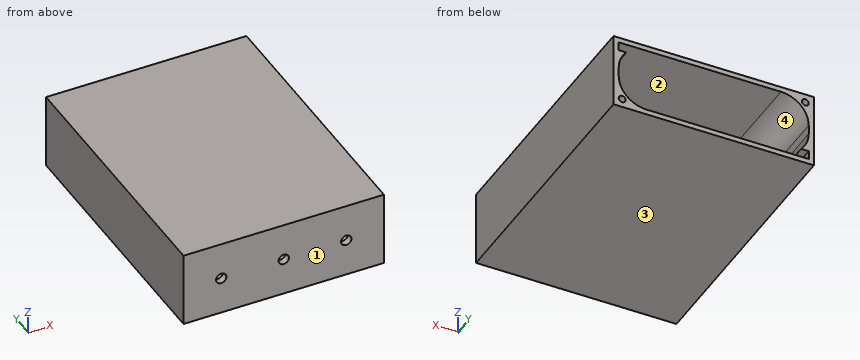
```python
from build123d import *

# Parameters (mm, degrees)
SKETCH1_W           = 57.7
SKETCH1_H           = 21.7
BOSS_EXTRUDE1_DEPTH = 2
SKETCH2_W           = 57.7
SKETCH2_H           = 21.7
SKETCH2_W_2         = 54.7
SKETCH2_H_2         = 18.7
BOSS_EXTRUDE2_DEPTH = 75
FILLET1_R           = 8
SKETCH3_W           = 38.583587397
SKETCH3_H           = 2.5
CUT_EXTRUDE1_DEPTH  = 75
SKETCH4_W           = 17.089400488
SKETCH4_H           = 2.5
CUT_EXTRUDE2_DEPTH  = 75
SKETCH5_R           = 1
CUT_EXTRUDE3_DEPTH  = 8
SKETCH6_R           = 1.5
CUT_EXTRUDE4_DEPTH  = 10


with BuildPart() as part:
    # Sketch1 → Boss-Extrude1 (new body)
    with BuildSketch(Plane(origin=(0, 0, 0), x_dir=(1, 0, 0), z_dir=(0, 1, 0))):
        with Locations((28.85, 10.85)):
            Rectangle(SKETCH1_W, SKETCH1_H)
    extrude(amount=BOSS_EXTRUDE1_DEPTH)

    # Sketch2 → Boss-Extrude2 (add)
    with BuildSketch(Plane(origin=(0, 2, 0), x_dir=(1, 0, 0), z_dir=(0, 1, 0))):
        with Locations((28.85, 10.85)):
            Rectangle(SKETCH2_W, SKETCH2_H)
        with Locations((28.85, 10.85)):
            Rectangle(SKETCH2_W_2, SKETCH2_H_2, mode=Mode.SUBTRACT)
    extrude(amount=BOSS_EXTRUDE2_DEPTH)

    # Fillet1
    fillet1_edges = [part.edges().sort_by_distance(p)[0] for p in [
        (1.5, 39.5, -20.2),
        (1.5, 39.5, -1.5),
        (56.2, 39.5, -1.5),
        (56.2, 39.5, -20.2),
    ]]
    fillet(fillet1_edges, radius=FILLET1_R)

    # Sketch3 → Cut-Extrude1 (cut)
    with BuildSketch(Plane(origin=(0, 77, 0), x_dir=(1, 0, 0), z_dir=(0, 1, 0))):
        with Locations((20.791793699, 18.95)):
            Rectangle(SKETCH3_W, SKETCH3_H)
    extrude(amount=-CUT_EXTRUDE1_DEPTH, mode=Mode.SUBTRACT)

    # Sketch4 → Cut-Extrude2 (cut)
    with BuildSketch(Plane(origin=(0, 77, 0), x_dir=(1, 0, 0), z_dir=(0, 1, 0))):
        with Locations((47.655299756, 2.75)):
            Rectangle(SKETCH4_W, SKETCH4_H)
    extrude(amount=-CUT_EXTRUDE2_DEPTH, mode=Mode.SUBTRACT)

    # Sketch5 → Cut-Extrude3 (cut)
    with BuildSketch(Plane(origin=(0, 77, 0), x_dir=(1, 0, 0), z_dir=(0, 1, 0))):
        with Locations(Location((55.2, 19.2, 0), (0, 0, 270))):
            Circle(SKETCH5_R)
        with Locations(Location((2.5, 2.5, 0), (0, 0, 270))):
            Circle(SKETCH5_R)
    extrude(amount=-CUT_EXTRUDE3_DEPTH, mode=Mode.SUBTRACT)

    # Sketch6 → Cut-Extrude4 (cut)
    with BuildSketch(Plane(origin=(0, 2, 0), x_dir=(1, 0, 0), z_dir=(0, 1, 0))):
        with Locations(Location((28.85, 10.85, 0), (0, 0, 270))):
            Circle(SKETCH6_R)
        with Locations(Location((10.85, 10.85, 0), (0, 0, 270))):
            Circle(SKETCH6_R)
        with Locations(Location((46.85, 10.85, 0), (0, 0, 270))):
            Circle(SKETCH6_R)
    extrude(amount=-CUT_EXTRUDE4_DEPTH, mode=Mode.SUBTRACT)


solid = part.part
```
The model under review builds one solid part; all positions refer to its coordinate system, in mm. Face numbers are marked on the shaded views. Round coordinates to 2 decimals unless told otherwise and drop trailing zeros. Order: outer loops, then holes, each group sorted by start corner. A loop starts at its lowest first (then second) coordinate and runs counter-clockwise, first axis right, second up.
Item 1: Add section A-A, the plane x = 28.85. State the section outline as (y, z) points.
Working result:
outline: (0, -21.7) - (77, -21.7) - (77, -20.2) - (2, -20.2) - (2, -12.35) - (0, -12.35) - close; (0, -9.35) - (2, -9.35) - (2, -1.5) - (77, -1.5) - (77, 0) - (0, 0) - close
Item 2: Add section C-C, the plane y = 33. State the section outline as (x, z) points.
Working result:
outline: (0, -21.7) - (57.7, -21.7) - (57.7, 0) - (0, 0) - close; hole (1.5, -20.2) - (48.2, -20.2) arc R8 ccw to (56.2, -12.2) - (56.2, -9.5) arc R8 ccw to (54.01, -4) - (56.2, -4) - (56.2, -1.5) - (9.5, -1.5) arc R8 ccw to (1.5, -9.5) - (1.5, -12.2) arc R8 ccw to (3.69, -17.7) - (1.5, -17.7) - close
Item 3: Add section D-D, the plane z = -14.75. State the section outline as (x, y) points.
Working result:
outline: (0, 0) - (57.7, 0) - (57.7, 77) - (55.78, 77) - (55.78, 2) - (1.92, 2) - (1.92, 77) - (0, 77) - close
Item 4: Draft analysis for pull direction Z (two halves, no side actions). For the marked faces 1, 2, 3 and 4, state which applies: released by +Z, released by -Z, zero draft, split by the parting line, or undercut.
Working result:
face 1: zero draft
face 2: undercut
face 3: released by -Z
face 4: undercut
Item 5: To check wall thickness, follow probe 1 along X at (y, z) = (1.65, -10.85); probe 2 along Z at (x, y) = (53.5, 23); probe 3 along Z at (x, y) = (42, 45). State the ranges of each line that lie inside material, in increasing order.
Working result:
probe 1: x = 0 to 9.35, 12.35 to 27.35, 30.35 to 45.35, 48.35 to 57.7
probe 2: z = -21.7 to -18.19, -1.5 to 0
probe 3: z = -21.7 to -20.2, -1.5 to 0
Item 6: Add section B-B, the plane z = -10.85. State the section outline as (x, y) points, and give its area (3 significant figures).
Working result:
outline: (0, 0) - (9.35, 0) - (9.35, 2) - (1.5, 2) - (1.5, 77) - (0, 77) - close; (12.35, 0) - (27.35, 0) - (27.35, 2) - (12.35, 2) - close; (30.35, 0) - (45.35, 0) - (45.35, 2) - (30.35, 2) - close; (48.35, 0) - (57.7, 0) - (57.7, 77) - (56.2, 77) - (56.2, 2) - (48.35, 2) - close
area: 322 mm2
Item 7: For pin 1 (2.5 mm diameter, centred on x = 10.85, z = -10.85, fed in from -Y); pin 2 (0.7 mm diameter, centred on x = 55, y = 31.5, fed in from +Z); pin 3 (0.6 mm diameter, centred on x = 2.5, z = -2.5, fed in from +Y); pin 4 (4 mm diameter, centred on x = 46.85, z = -10.85, fed in from +Y), all flat-tipped, find the tip position at first contact; note any pin that passes through.
Working result:
pin 1: passes through
pin 2: stops at z = 0
pin 3: stops at y = 69
pin 4: stops at y = 2
